```python
from build123d import *

# Parameters (mm, degrees)
F0_R     = 16
F1_DEPTH = 3
F2_R     = 8
F3_DEPTH = 10
F4_R     = 4
F5_DEPTH = 13.001
F6_R     = 2
F7_DEPTH = 3.001
F8_SIZE  = 0.5


with BuildPart() as f1:
    # F0 (on Front) → F1 (new body)
    with BuildSketch(Plane.XZ):
        Circle(F0_R)
    extrude(amount=F1_DEPTH)

    # F2 (on face) → F3 (join)
    with BuildSketch(Plane.XZ.offset(3)):
        Circle(F2_R)
    extrude(amount=F3_DEPTH)

    # F4 (on face) → F5 (cut, through all)
    with BuildSketch(Plane.XZ.offset(13)):
        Circle(F4_R)
    extrude(amount=-F5_DEPTH, mode=Mode.SUBTRACT)

    # F6 (on face) → F7 (cut, through all)
    with BuildSketch(Plane.XZ.offset(3)):
        with Locations((0, 12)):
            Circle(F6_R)
        with Locations((-12, 0)):
            Circle(F6_R)
        with Locations((0, -12)):
            Circle(F6_R)
        with Locations((12, 0)):
            Circle(F6_R)
    extrude(amount=-F7_DEPTH, mode=Mode.SUBTRACT)

    # F8
    f8_edges = [f1.edges().sort_by_distance(p)[0] for p in [
        (-8, -13, 0),
        (-4, -13, 0),
        (-16, 0, 0),
        (-2, 0, -12),
        (-14, 0, 0),
        (-4, 0, 0),
        (10, 0, 0),
        (-2, 0, 12),
        (-16, -3, 0),
        (-2, -3, 12),
        (-14, -3, 0),
        (10, -3, 0),
        (-2, -3, -12),
    ]]
    chamfer(f8_edges, length=F8_SIZE)


solid = f1.part
```
For this review, take the finished solid that the model builds, in its own axes (mm). Give positions to 0.01 mm unless a question says otherwise; leave off trailing zeros. Write each loop counter-clockwise with the first axis right and the second up, starting at its lowest first coordinate (ties: lowest second). Pieces come first, ordered by that corner, then holes.
Item 1: Take a section at A-A (y = -9). Give the boundary of the cut face in (x, z).
Item 2: The part is to be moulded in two halves that separate along X. For faces 1 (the face through (10.4, -1.5, -1.2)), 2 (the face through (0, -2, -10)), 3 (the face through (7, -3, -7)), 4 (the face through (-1.73, -7.68, -7.81)), say which applies: +X half, -X half, draft (parallel to the pull), parting line (faces both ways), or undercut.
Item 3: Take a section at D-D (y = -1.5). Give the boundary of the cut face in (x, z), and give its area (3 significant figures).
Item 4: Insertion check: P1, Ø6.5, axis at x = 0, z = -12, coming from the -Y side; P2, Ø4.5, axis at x = 12, z = 0, coming from the -Y side; P3, Ø3, axis at y = -8.5, z = 7, coming from the +X side; P4, Ø5, axis at x = -11.5, y = -9, coming from the -Z side. Each pin has a flat end and moves straight along its axis. Give the tip position at first contact, or say it passes through.
Item 5: Take a section at B-B (x = 0). Give the number of separate pieces and of enclosed holes in the cut face, and give its area (3 significant figures).
Item 6: Wall thickness on probe 1 along Z at (x, y) = (0, -1.9); probe 2 along Z at (x, y) = (0, -3.5); probe 3 along X at (y, z) = (-2.5, -0.5): over which ranges is each line inside the solid? List them lowest first.
Established:
1. outline: circle Ø16 at (0, 0); hole circle Ø8 at (0, 0)
2. face 1: undercut
2. face 2: undercut
2. face 3: draft
2. face 4: parting line
3. outline: circle Ø32 at (0, 0); hole circle Ø4 at (-12, 0); hole circle Ø8 at (0, 0); hole circle Ø4 at (0, -12); hole circle Ø4 at (0, 12); hole circle Ø4 at (12, 0)
3. area: 704 mm2
4. P1: stops at y = -3
4. P2: stops at y = -2.75
4. P3: stops at x = 5.81
4. P4: passes through
5. separate pieces: 4
5. enclosed holes: 0
5. area: 126 mm2
6. probe 1: z = -16 to -14, -10 to -4, 4 to 10, 14 to 16
6. probe 2: z = -8 to -4, 4 to 8
6. probe 3: x = -15.99 to -13.94, -10.06 to -3.97, 3.97 to 10.06, 13.94 to 15.99
